Read the model definition and answer for the solid it produces. Units are mm, in the model's axes. Round coordinates to 2 decimals unless told otherwise and drop trailing zeros. Write each loop counter-clockwise with the first axis right and the second up, starting at its lowest first coordinate (ties: lowest second). Pieces come first, ordered by that corner, then holes. Notation, with made-up numbers: (35, -5) - (83, -5) arc R8 ccw to (83, 5) - close; hole circle Ø1 at (75, -14). An arc over 180 degrees is marked (long way). One line per item, written item: value. Start each with the question number.
(1) A cutting plane is placed at B-B, the plane x = 176.5. Determine the outline of the cut face in (y, z), plus the area to 3 significant figures.
(2) A cutting plane is placed at D-D, the plane x = 216. Determine the outline of the cut face in (y, z), plus the area to 3 significant figures.
(3) A cutting plane is placed at A-A, the plane z = 26. Determine the outline of the cut face in (x, y), plus the area to 3 significant figures.
(4) Find the intervals of material crossed by L1, parallel to X at y = 1.75, z = -54; L2, parallel to X at y = 3.95, z = 22; L3, parallel to X at y = 0.75, z = 6, in increasing order.
(5) Flat-ended cylindrical pins translate along their axes: pin 1 Ø11.5 at (x, z) = (114.3, -54.356) entering from -Y; pin 2 Ø5 at (x, z) = (151.64, 5.46) entering from -Y; pin 3 Ø2 at (y, z) = (4, 12) entering from -X; pin 4 Ø3 at (y, z) = (3.5, 16.5) entering from -X. Find the tip coordinate at first contact, or state that the pin passes through.
(6) A cutting plane is placed at C-C, the plane y = 3. State how many separate pieces and enclosed holes the cut face has, plus the area to 3 significant figures.
from build123d import *

# Parameters (mm, degrees)
BOSS_EXTRUDE1_DEPTH   = 5.588
F_6_CLEARANCE_HOLE1_D = 3.7973
CUT_EXTRUDE1_REACH    = 254.133
SKETCH5_R             = 5.08
CUT_EXTRUDE2_REACH    = 254.133
SKETCH6_R             = 6.35
CUT_EXTRUDE3_REACH    = 254.133
SKETCH7_R             = 2.54


with BuildPart() as part:
    # Sketch1 → Boss-Extrude1 (new body)
    with BuildSketch(Plane(origin=(0, 0, 0), x_dir=(1, 0, 0), z_dir=(0, 1, 0))):
        with BuildLine():
            Line((12.7, 72.898), (31.75, 72.898))
            Line((31.75, 72.898), (31.75, 67.056))
            Line((31.75, 67.056), (44.45, 67.056))
            Line((44.45, 67.056), (44.45, 72.898))
            Line((44.45, 72.898), (69.85, 72.898))
            Line((69.85, 72.898), (69.85, 67.31))
            Line((69.85, 67.31), (114.3, 67.31))
            Line((114.3, 67.31), (114.3, 72.898))
            Line((114.3, 72.898), (139.7, 72.898))
            Line((139.7, 72.898), (139.7, 67.31))
            Line((139.7, 67.31), (165.1, 67.31))
            Line((165.1, 67.31), (165.1, 72.898))
            Line((165.1, 72.898), (190.5, 72.898))
            Line((190.5, 72.898), (190.5, 67.056))
            Line((190.5, 67.056), (222.25, 67.056))
            Line((222.25, 67.056), (222.25, 72.898))
            Line((222.25, 72.898), (241.3, 72.898))
            Line((241.3, 72.898), (241.3, 0))
            Line((241.3, 0), (171.45, 0))
            ThreePointArc((171.45, 0), (162.469743879, -3.719743879), (158.75, -12.7))
            Line((158.75, -12.7), (158.75, -42.164))
            Line((158.75, -42.164), (146.05, -42.164))
            Line((146.05, -42.164), (146.05, 0.122766638))
            Line((146.05, 0.122766638), (127, 0.122766638))
            Line((127, 0.122766638), (107.95, 0.122766638))
            Line((107.95, 0.122766638), (107.95, -42.164))
            Line((107.95, -42.164), (95.25, -42.164))
            Line((95.25, -42.164), (95.25, -12.7))
            ThreePointArc((95.25, -12.7), (91.530256121, -3.719743879), (82.55, 0))
            Line((82.55, 0), (12.7, 0))
            Line((12.7, 0), (12.7, 72.898))
        make_face()
    extrude(amount=BOSS_EXTRUDE1_DEPTH)

    # #6 Clearance Hole1 (through all)
    with Locations(Plane(origin=(0, 0, 0), x_dir=(-1, 0, 0), z_dir=(0, -1, 0))):
        with Locations((-102.362, -32.397617544), (-151.638, -32.397617544), (-151.638, -5.456849181), (-102.362, -5.456849181)):
            Hole(F_6_CLEARANCE_HOLE1_D / 2)

    # Sketch5 → Cut-Extrude1 (cut, up to next)
    with BuildSketch(Plane(origin=(0, 5.588, 0), x_dir=(1, 0, 0), z_dir=(0, 1, 0)), mode=Mode.PRIVATE) as cut_extrude1_sk1:
        with Locations(Location((225.552, 15.870766638, 0), (0, 0, 270))):
            Circle(SKETCH5_R)
    cut_extrude1_tool1 = extrude(cut_extrude1_sk1.sketch, amount=-CUT_EXTRUDE1_REACH, mode=Mode.PRIVATE) & part.part
    # Sketch5 → Cut-Extrude1 (cut, up to next)
    with BuildSketch(Plane(origin=(0, 5.588, 0), x_dir=(1, 0, 0), z_dir=(0, 1, 0)), mode=Mode.PRIVATE) as cut_extrude1_sk2:
        with Locations(Location((28.448, 15.870766638, 0), (0, 0, 270))):
            Circle(SKETCH5_R)
    cut_extrude1_tool2 = extrude(cut_extrude1_sk2.sketch, amount=-CUT_EXTRUDE1_REACH, mode=Mode.PRIVATE) & part.part
    add(cut_extrude1_tool1.solids().sort_by_distance((225.552, 5.588, -15.870767))[0], mode=Mode.SUBTRACT)
    add(cut_extrude1_tool2.solids().sort_by_distance((28.448, 5.588, -15.870767))[0], mode=Mode.SUBTRACT)

    # Sketch6 → Cut-Extrude2 (cut, up to next)
    with BuildSketch(Plane.XZ, mode=Mode.PRIVATE) as cut_extrude2_sk1:
        with Locations(Location((114.3, -54.356, 0), (0, 0, 270))):
            Circle(SKETCH6_R)
    cut_extrude2_tool1 = extrude(cut_extrude2_sk1.sketch, amount=-CUT_EXTRUDE2_REACH, mode=Mode.PRIVATE) & part.part
    add(cut_extrude2_tool1.solids().sort_by_distance((114.3, 0, -54.356))[0], mode=Mode.SUBTRACT)

    # Sketch7 → Cut-Extrude3 (cut, up to next)
    with BuildSketch(Plane(origin=(0, 5.588, 0), x_dir=(1, 0, 0), z_dir=(0, 1, 0)), mode=Mode.PRIVATE) as cut_extrude3_sk1:
        with Locations(Location((139.7, 54.020508314, 0), (0, 0, 270))):
            Circle(SKETCH7_R)
    cut_extrude3_tool1 = extrude(cut_extrude3_sk1.sketch, amount=-CUT_EXTRUDE3_REACH, mode=Mode.PRIVATE) & part.part
    # Sketch7 → Cut-Extrude3 (cut, up to next)
    with BuildSketch(Plane(origin=(0, 5.588, 0), x_dir=(1, 0, 0), z_dir=(0, 1, 0)), mode=Mode.PRIVATE) as cut_extrude3_sk2:
        with Locations(Location((88.9, 54.020508314, 0), (0, 0, 270))):
            Circle(SKETCH7_R)
    cut_extrude3_tool2 = extrude(cut_extrude3_sk2.sketch, amount=-CUT_EXTRUDE3_REACH, mode=Mode.PRIVATE) & part.part
    add(cut_extrude3_tool1.solids().sort_by_distance((139.7, 5.588, -54.020508))[0], mode=Mode.SUBTRACT)
    add(cut_extrude3_tool2.solids().sort_by_distance((88.9, 5.588, -54.020508))[0], mode=Mode.SUBTRACT)


solid = part.part
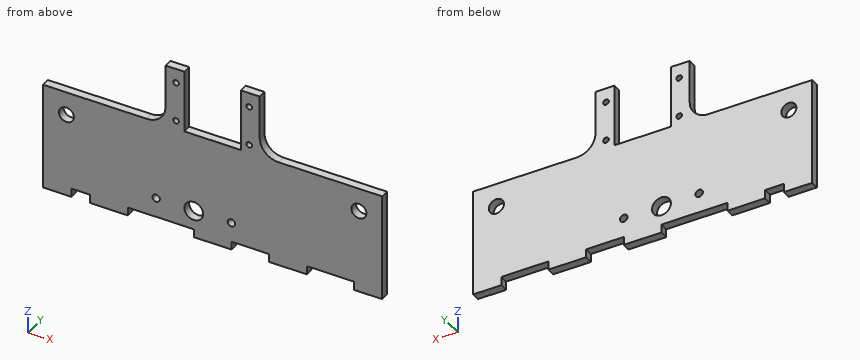
Here are the results:
1. outline: (0, -72.9) - (5.59, -72.9) - (5.59, 0) - (0, 0) - close
1. area: 407 mm²
2. outline: (0, -67.06) - (5.59, -67.06) - (5.59, 0) - (0, 0) - close
2. area: 375 mm²
3. outline: (95.25, 0) - (107.95, 0) - (107.95, 5.59) - (95.25, 5.59) - close; (146.05, 0) - (158.75, 0) - (158.75, 5.59) - (146.05, 5.59) - close
3. area: 142 mm²
4. L1: 12.7 to 86.36, 91.44 to 107.96, 120.64 to 137.16, 142.24 to 241.3
4. L2: 95.25 to 107.95, 146.05 to 158.75
4. L3: 93.34 to 100.54, 104.18 to 107.95, 146.05 to 149.82, 153.46 to 160.66
5. pin 1: through
5. pin 2: y = 0
5. pin 3: x = 95.14
5. pin 4: x = 95.25
6. separate pieces: 1
6. enclosed holes: 9
6. area: 16,800 mm²
